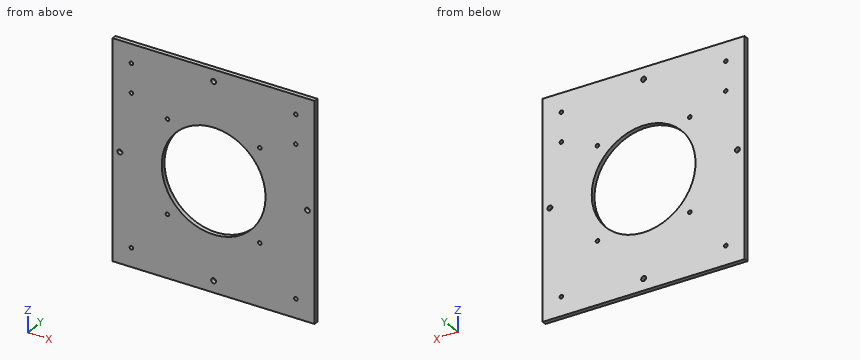
```python
from build123d import *

# Parameters (mm, degrees)
SKETCH_1_W           = 140
SKETCH_1_H           = 3
EXTRUDE_1_DEPTH      = 150
CUT_EXTRUDE_1_REACH  = 5
SKETCH_2_R           = 36
HOLE_WIZARD_M3_1_D   = 2.5
HOLE_WIZARD_M3_1_2_D = 3.4
HOLE_WIZARD_M3_2_D   = 2.5


with BuildPart() as part:
    # 草图1 → 拉伸-薄壁1 (new body)
    with BuildSketch(Plane.XY):
        with Locations((82, 225.557982809)):
            Rectangle(SKETCH_1_W, SKETCH_1_H)
    extrude(amount=EXTRUDE_1_DEPTH)

    # 草图2 → 切除-拉伸1 (cut, up to next)
    with BuildSketch(Plane.XZ.offset(-224.057982809), mode=Mode.PRIVATE) as cut_extrude_1_sk1:
        with Locations((82, 75)):
            Circle(SKETCH_2_R)
    cut_extrude_1_tool1 = extrude(cut_extrude_1_sk1.sketch, amount=-CUT_EXTRUDE_1_REACH, mode=Mode.PRIVATE) & part.part
    add(cut_extrude_1_tool1.solids().sort_by_distance((82, 224.057983, 75))[0], mode=Mode.SUBTRACT)

    # Hole Wizard M3 _1 (through all)
    with Locations(Plane(origin=(0, 224.057982809, 0), x_dir=(-1, 0, 0), z_dir=(0, -1, 0))):
        with Locations((-50, -107), (-50, -43), (-114, -43), (-114, -107)):
            Hole(HOLE_WIZARD_M3_1_D / 2)

    # Hole Wizard M3 _1 2 (through all)
    with Locations(Plane(origin=(0, 224.057982809, 0), x_dir=(-1, 0, 0), z_dir=(0, -1, 0))):
        with Locations((-82, -142), (-147, -75), (-82, -8), (-17, -75)):
            Hole(HOLE_WIZARD_M3_1_2_D / 2)

    # M3 螺纹孔的螺纹孔钻头2 (through all)
    with Locations(Plane(origin=(0, 224.057982809, 0), x_dir=(-1, 0, 0), z_dir=(0, -1, 0))):
        with Locations((-139, -137), (-139, -117), (-139, -13), (-25, -137), (-25, -117), (-25, -13)):
            Hole(HOLE_WIZARD_M3_2_D / 2)


solid = part.part
```
Work out the finished part from the listing and answer in its coordinate system (mm). Coordinates: 2 decimals unless noted, no trailing zeros. Write each loop counter-clockwise with the first axis right and the second up, starting at its lowest first coordinate (ties: lowest second). Pieces come first, ordered by that corner, then holes. Notation, with made-up numbers: (76, 56.5) - (103, 56.5) arc R31 cw to (103, 88.5) - close; hole circle Ø2 at (3, -23.5). An arc over 180 degrees is marked (long way). Answer as a JSON object with one key per item and string values.
Q1. Given pin 1 Ø2 at (x, z) = (114, 107) entering from +Y; pin 2 Ø3 at (x, z) = (139, 13) entering from -Y, each flat-ended and moving along its own axis, determine where each tip first touches the part or whether it passes through.
Results list:
{"pin 1": "passes through", "pin 2": "stops at y = 224.06"}
Q2. Find section B-B (x = 17). Write down the section's boundary in (y, z), plus the area to 3 significant figures.
Results list:
{"outline": "(224.06, 0) - (227.06, 0) - (227.06, 73.3) - (224.06, 73.3) - close; (224.06, 76.7) - (227.06, 76.7) - (227.06, 150) - (224.06, 150) - close", "area": "440 mm^2"}
Q3. Find section A-A (z = 8). Write down the section's boundary in (x, y).
Results list:
{"outline": "(12, 224.06) - (80.3, 224.06) - (80.3, 227.06) - (12, 227.06) - close; (83.7, 224.06) - (152, 224.06) - (152, 227.06) - (83.7, 227.06) - close"}
Q4. Consider L1, parallel to Z at x = 82, y = 226.1; L2, parallel to X at y = 225.1, z = 13; L3, parallel to Z at x = 25, y = 225.5. Determine where each line is inside the solid, lowest interval first. Write a range as from..to.
Results list:
{"L1": "z = 0..6.3, 9.7..39, 111..140.3, 143.7..150", "L2": "x = 12..23.75, 26.25..137.75, 140.25..152", "L3": "z = 0..11.75, 14.25..115.75, 118.25..135.75, 138.25..150"}
Q5. Find section C-C (y = 226.55). State how many separate pieces and enclosed holes the cut face has, plus the area to 3 significant figures.
Results list:
{"separate pieces": "1", "enclosed holes": "15", "area": "16,800 mm^2"}
